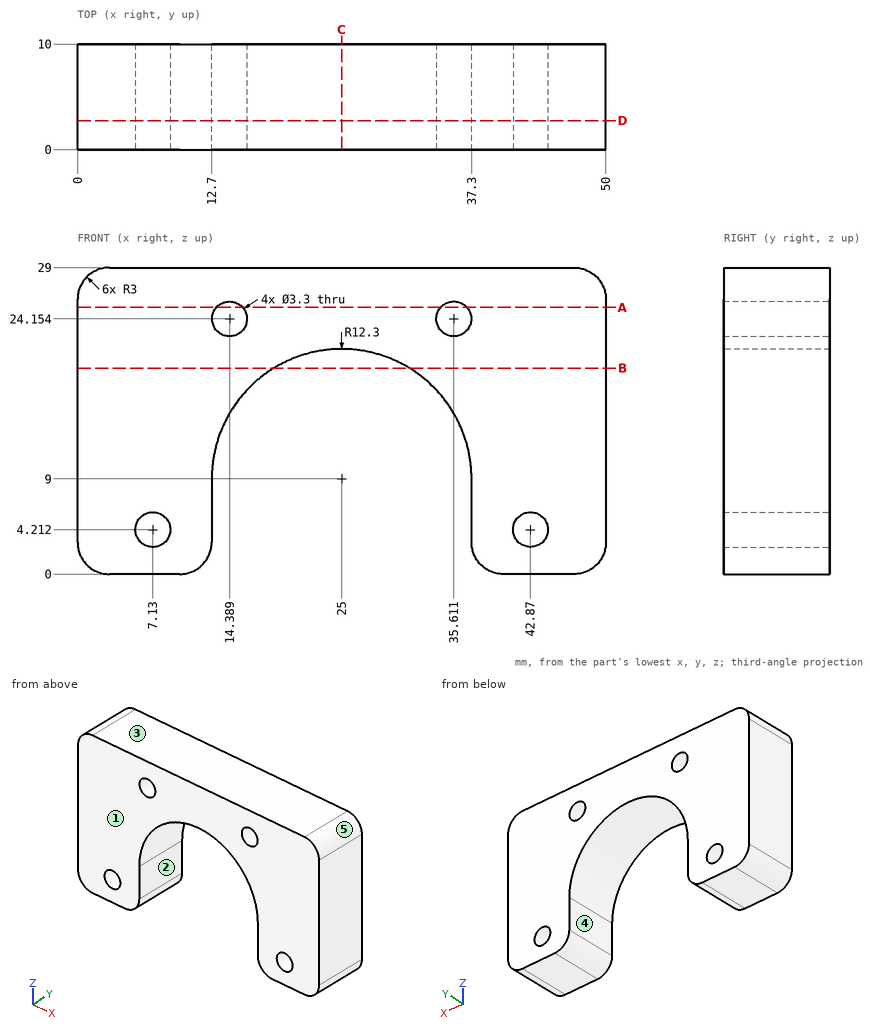
The drawing under review shows one solid part. Ordinate dimensions are in mm from its lowest x, y, z. A direction names the side the tool comes from. Round coordinates to 2 decimals unless told otherwise and drop trailing zeros. Loops run counter-clockwise (first coordinate to the right, second up) from the corner with the lowest first, then second, coordinate; pieces in that order, holes last. Notation, with made-up numbers: (76.25, 21) -> (129.25, 21) arc R7 cw to (129.25, 31) -> close; hole circle Ø4 at (-11, 16). An arc over 180 degrees is marked (long way). Answer in a Markdown table with one row per item.
1) Consider section A-A, the plane z = 25.25. Write out the cut boundary in (x, y) (1 decimal).
Taken from the geometry:
| item | result |
|---|---|
| outline | (0, 0) -> (13.2, 0) -> (13.2, 10) -> (0, 10) -> close; (15.6, 0) -> (34.4, 0) -> (34.4, 10) -> (15.6, 10) -> close; (36.8, 0) -> (50, 0) -> (50, 10) -> (36.8, 10) -> close |
2) Draft analysis for pull direction X (two halves, no side actions). For the marked faces 3, 4 and 5, state which applies: pulls with the +X half, pulls with the -X half, needs draft (parallel to the pull), parting line crosses it, or undercut.
Taken from the geometry:
| item | result |
|---|---|
| face 3 | needs draft |
| face 4 | undercut |
| face 5 | pulls with the +X half |
3) For pin 1 Ø3 at (x, z) = (7.13, 4.21) entering from -Y, flat-tipped, find the tip position at first contact; note if it passes through.
Taken from the geometry:
| item | result |
|---|---|
| pin 1 | passes through |
4) Wall thickness on line 1 along X through (y, z) = (6.25, 6.75); line 2 along Z through (x, y) = (43, 0.5); line 3 along X through (y, z) = (4.75, 3.5): over which ranges is each line inside the solid? List them lowest first.
Taken from the geometry:
| item | result |
|---|---|
| line 1 | x = 0 to 12.7, 37.3 to 50 |
| line 2 | z = 0 to 2.57, 5.86 to 29 |
| line 3 | x = 0 to 5.64, 8.62 to 12.7, 37.3 to 41.38, 44.36 to 50 |
5) Consider section C-C, the plane x = 25. Write out the cut boundary in (y, z).
Taken from the geometry:
| item | result |
|---|---|
| outline | (0, 21.3) -> (10, 21.3) -> (10, 29) -> (0, 29) -> close |
6) Consider section D-D, the plane y = 2.75. Count the separate pieces of the cut face and the enclosed holes in it, plus the area to 3 significant figures.
Taken from the geometry:
| item | result |
|---|---|
| separate pieces | 1 |
| enclosed holes | 4 |
| area | 945 mm² |
7) Consider section B-B, the plane z = 19.5. Write out the cut boundary in (x, y), plus the area to 3 significant figures.
Taken from the geometry:
| item | result |
|---|---|
| outline | (0, 0) -> (18.59, 0) -> (18.59, 10) -> (0, 10) -> close; (31.41, 0) -> (50, 0) -> (50, 10) -> (31.41, 10) -> close |
| area | 372 mm² |
8) Tool access review of the marked faces 1 and 2: name each direction out of +Z, -Z, +X, -X, +Y, -Y from which nothing blocks a thin tool from reaching the whole face with its end or side.
Taken from the geometry:
| item | result |
|---|---|
| face 1 | +Z, -Z, +X, -X, -Y |
| face 2 | -Z, +Y, -Y |
